Part print with two shaded views. Sizes in mm from the minimum x, y, z corner. A direction names the side the tool comes from. Round coordinates to 2 decimals unless told otherwise and drop trailing zeros. Order: outer loops, then holes, each group sorted by start corner. A loop starts at its lowest first (then second) coordinate and runs counter-clockwise, first axis right, second up. Notation, with made-up numbers: (-34.75, 87.5) -> (-12.75, 87.5) arc R7 cw to (-12.75, 94.5) -> close; hole circle Ø4 at (87, 49.25). An arc over 180 degrees is marked (long way). Put each result on its own line as item: value. Start each with the question number.
Q1. 3-axis set-ups, long thin cutter, end or side, ignore diameter. For the marked faces 1 and 2: which of +Z, -Z, +X, -X, +Y, -Y reach the whole face in a straight line?
Q2. Probe L1, parallel to Z at x = 29, y = 4.5 (1 decimal); L2, parallel to Z at x = 28, y = 5.25 (1 decimal); L3, parallel to Y at x = 28, z = 32. List the from-to ranges inside material, lowest first.
Q3. Cut at A-A, the plane x = 27.5. List the corners of the cut face in (y, z), and give its area (3 significant figures).
Q4. Cut at D-D, the plane x = 20.5. List the corners of the cut face in (y, z) (1 decimal).
Q5. Pull direction X, two halves, no side cores. Call the marked faces 3, 4 and 5: released by +X, released by -X, zero draft, split by the parting line, or undercut.
Q6. Cut at C-C, the plane y = 7. List the corners of the cut face in (x, z) (1 decimal), and give its area (3 significant figures).
Q7. Flat gauge pins, fed straight in: P1, Ø2, axis at x = 43, y = 8.5, coming from the -Z side; P2, Ø6, axis at x = 30, y = 5.5, coming from the -Z side; P3, Ø1.5, axis at x = 41.5, y = 4.5, coming from the -Z side. Where does each tip first touch, or does it go through?
Q8. Cut at B-B, the plane z = 8. List the corners of the cut face in (x, y).
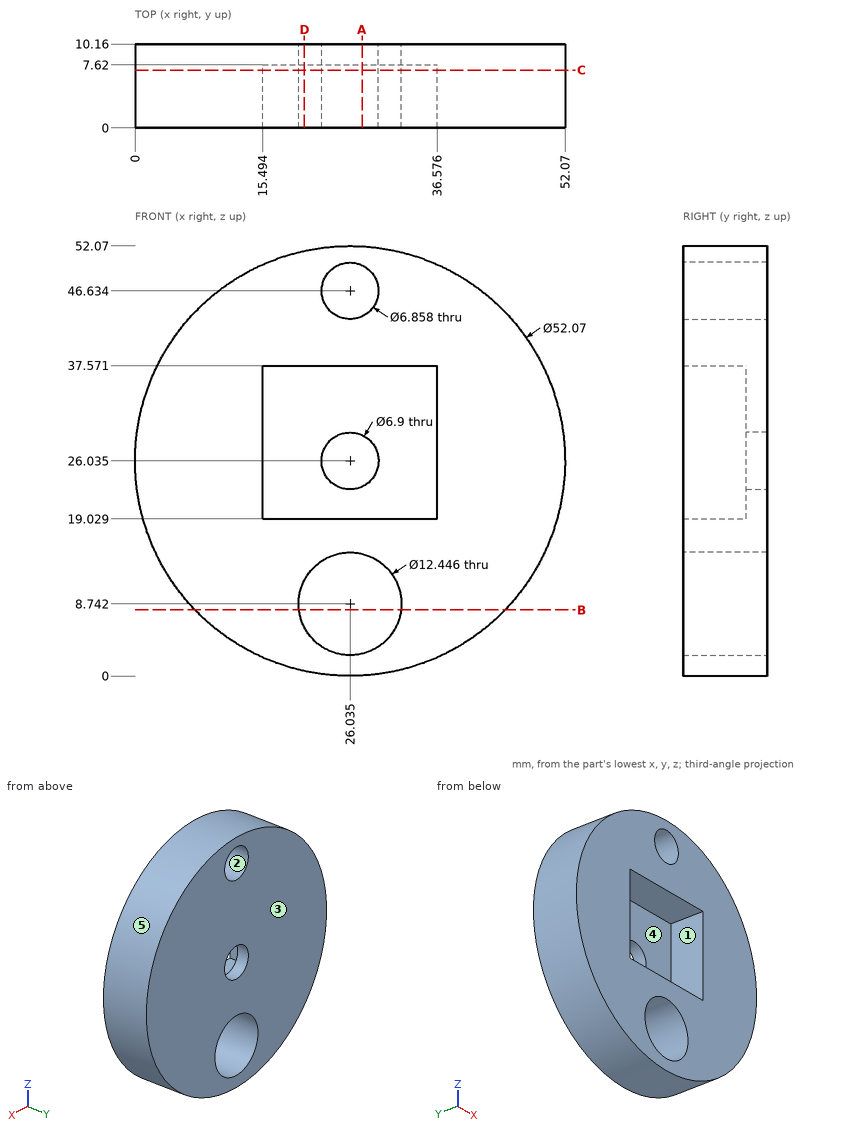
Ans:
1. face 1: -Y
1. face 2: +Y, -Y
2. L1: z = 0.2 to 3.3, 14.2 to 19, 37.6 to 44.9, 48.4 to 51.9
2. L2: z = 0.1 to 2.8, 14.6 to 19, 37.6 to 43.8, 49.4 to 52
2. L3: y = 7.62 to 10.16
3. outline: (0, 0.04) -> (10.16, 0.04) -> (10.16, 2.69) -> (0, 2.69) -> close; (0, 14.79) -> (10.16, 14.79) -> (10.16, 22.91) -> (7.62, 22.91) -> (7.62, 19.03) -> (0, 19.03) -> close; (0, 37.57) -> (7.62, 37.57) -> (7.62, 29.16) -> (10.16, 29.16) -> (10.16, 43.53) -> (0, 43.53) -> close; (0, 49.73) -> (10.16, 49.73) -> (10.16, 52.03) -> (0, 52.03) -> close
3. area: 185 mm^2
4. outline: (0, 0.6) -> (10.2, 0.6) -> (10.2, 5.9) -> (0, 5.9) -> close; (0, 11.6) -> (10.2, 11.6) -> (10.2, 51.5) -> (0, 51.5) -> (0, 37.6) -> (7.6, 37.6) -> (7.6, 19) -> (0, 19) -> close
5. face 3: zero draft
5. face 4: undercut
5. face 5: split by the parting line
6. outline: circle Ø52.1 at (26, 26); hole (15.5, 19) -> (36.6, 19) -> (36.6, 37.6) -> (15.5, 37.6) -> close; hole circle Ø12.4 at (26, 8.7); hole circle Ø6.9 at (26, 46.6)
6. area: 1,580 mm^2
7. P1: stops at z = 5.47
7. P2: stops at z = 0.02
7. P3: stops at z = 4.56
8. outline: (7.26, 0) -> (19.86, 0) -> (19.86, 10.16) -> (7.26, 10.16) -> close; (32.21, 0) -> (44.81, 0) -> (44.81, 10.16) -> (32.21, 10.16) -> close
